CAD build for the part. Positions are in the model's coordinates, mm. Coordinates: 2 decimals unless noted, no trailing zeros. Order: outer loops, then holes, each group sorted by start corner. A loop starts at its lowest first (then second) coordinate and runs counter-clockwise, first axis right, second up. Notation, with made-up numbers: M 79,-19 L 101,-19 A32 cw 101,15 Z; hole C 55.5,-23.5 d8. An arc over 180 degrees is marked long. One line per item, written item: value.
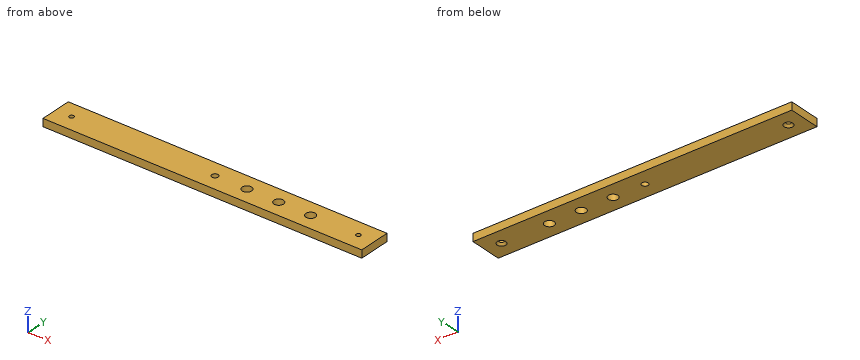
Solid Edge part; units mm, degrees
sketch "Sketch1" plane through (0, 0, 0) normal (0, 0, 1) x (1, 0, 0)
  line L0 (250, -25) -> (-250, -25)
  line L1 (-250, -25) -> (-250, 25)
  line L2 (-250, 25) -> (250, 25)
  line L3 (250, 25) -> (250, -25)
extrude "Protrusion1" add sketch "Sketch1" against normal blind 12
hole "Hole_2" at (-225, 0, -12) direction (0, 0, 1) diameter 7 end up to next countersink diameter 13.71 countersink angle 90
hole "Hole1" at (225, 0, -12) direction (0, 0, 1) diameter 7 end up to next countersink diameter 13.71 countersink angle 90
hole "Hole_3" at (0, 0, -12) direction (0, 0, 1) diameter 10 end up to next
hole "Hole_4" at (150, 0, -12) direction (0, 0, 1) diameter 15 end up to next
hole "Hole2" at (100, 0, -12) direction (0, 0, 1) diameter 15 end up to next
hole "Hole3" at (50, 0, -12) direction (0, 0, 1) diameter 15 end up to next
Q1. Slice it at B-B (z = -6.5). List the corners of the cut face in (x, y), plus the area to 3 significant figures.
Recorded:
outline: M -250,-25 L 250,-25 L 250,25 L -250,25 Z; hole C -225,0 d7; hole C 0,0 d10; hole C 50,0 d15; hole C 100,0 d15; hole C 150,0 d15; hole C 225,0 d7
area: 24,300 mm^2
Q2. Drill centre lines: line 1 along Y through (x, z) = (150, -5.25); line 2 along Y through (x, z) = (-225, -6.25). Where is each one in solid material? Low to high.
Recorded:
line 1: y = -25 to -7.5, 7.5 to 25
line 2: y = -25 to -3.5, 3.5 to 25
Q3. Slice it at C-C (x = 50). List the corners of the cut face in (y, z), plus the area to 3 significant figures.
Recorded:
outline: M -25,-12 L -7.5,-12 L -7.5,0 L -25,0 Z; M 7.5,-12 L 25,-12 L 25,0 L 7.5,0 Z
area: 420 mm^2
Q4. Pin check, flat tips, straight feed: pin 1 Ø6.5 at (x, y) = (225, 0) entering from +Z; pin 2 Ø11 at (x, y) = (-225, 0) entering from -Z (3 decimals). Stop position of each tip, or through.
Recorded:
pin 1: passes through
pin 2: stops at z = -10.645
Q5. Slice it at A-A (x = 0). List the corners of the cut face in (y, z).
Recorded:
outline: M -25,-12 L -5,-12 L -5,0 L -25,0 Z; M 5,-12 L 25,-12 L 25,0 L 5,0 Z
